Part model, mm, in its own coordinate system. A direction names the side the tool comes from. Coordinates: 2 decimals unless noted, no trailing zeros. Loops run counter-clockwise (first coordinate to the right, second up) from the corner with the lowest first, then second, coordinate; pieces in that order, holes last. Notation, with made-up numbers: M -15,36.5 L 28,36.5 A15 ccw 28,48.5 Z; hole C 33,24 d9. An arc over 180 degrees is marked long. Use a Markdown table: item, result. Add a question column.
1) Band-saw the part on C-C (x = -18.5). List the corners of the cut face in (y, z), plus the area to 3 significant figures.
2) Pull direction Z, two halves, no side cores. Call faces 5 (the flat face through (0, 1.2, 0)), 6 (the flat face through (22.5, 10, 0)), 7 (the flat face through (-11.5, 12, -23)): released by +Z, released by -Z, zero draft, split by the parting line, or undercut.
3) Band-saw the part on D-D (z = -0.5). List the corners of the cut face in (x, y), plus the area to 3 significant figures.
4) Band-saw the part on A-A (y = 13). List the corners of the cut face in (x, z).
5) Pin check, flat tips, straight feed: pin 1 Ø0.7 at (x, z) = (18.5, -18.5) entering from +Y; pin 2 Ø3 at (x, z) = (-18, -17.5) entering from +Y; pin 3 Ø1.3 at (x, z) = (-0.5, -23) entering from +Y. Stop position of each tip, or through.
6) Tool access for faces 1 (the cylindrical face through (-17.806, 3.721, 18.409)), 2 (the flat face through (-23, 12, 2)), 3 (the flat face through (11.5, 12, -23)), 4 (the flat face through (-9, 6.2, 23)): list every direction of +Z, -Z, +X, -X, +Y, -Y with a clear straight run to the whole face (end or side of a thin tool).
7) Band-saw the part on B-B (z = 10.5). List the corners of the cut face in (x, y).
8) Wall check: probe 1 along X at (y, z) = (3.6, -18.5); probe 2 along X at (y, z) = (4.75, -19); probe 3 along Z at (x, y) = (15, 15.25). Give the ranges that are in metal, low to high. Write a range as from..to.
from build123d import *

# Parameters (mm, degrees)
SKETCH1_W           = 47.4
SKETCH1_H           = 47.4
BOSS_EXTRUDE1_DEPTH = 18
SKETCH2_W           = 45
SKETCH2_H           = 45
CUT_EXTRUDE1_DEPTH  = 16.8
SKETCH3_R           = 1.75
BOSS_EXTRUDE2_DEPTH = 4
SKETCH4_R           = 0.7
CUT_EXTRUDE2_DEPTH  = 3
SKETCH5_W           = 16
SKETCH5_H           = 1.2
SKETCH5_W_2         = 1.2
SKETCH5_H_2         = 10.5
SKETCH5_W_3         = 23
CUT_EXTRUDE3_DEPTH  = 11.8


with BuildPart() as part:
    # Sketch1 → Boss-Extrude1 (new body)
    with BuildSketch(Plane(origin=(0, 0, 0), x_dir=(1, 0, 0), z_dir=(0, 1, 0))):
        Rectangle(SKETCH1_W, SKETCH1_H)
    extrude(amount=BOSS_EXTRUDE1_DEPTH)

    # Sketch2 → Cut-Extrude1 (cut)
    with BuildSketch(Plane(origin=(0, 18, 0), x_dir=(1, 0, 0), z_dir=(0, 1, 0))):
        Rectangle(SKETCH2_W, SKETCH2_H)
    extrude(amount=-CUT_EXTRUDE1_DEPTH, mode=Mode.SUBTRACT)

    # Sketch3 → Boss-Extrude2 (add)
    with BuildSketch(Plane(origin=(0, 1.2, 0), x_dir=(1, 0, 0), z_dir=(0, 1, 0))):
        with Locations(Location((-18.5, 18.5, 0), (0, 0, 270))):
            Circle(SKETCH3_R)
        with Locations(Location((18.5, 18.5, 0), (0, 0, 270))):
            Circle(SKETCH3_R)
        with Locations(Location((18.5, -18.5, 0), (0, 0, 270))):
            Circle(SKETCH3_R)
        with Locations(Location((-18.5, -18.5, 0), (0, 0, 270))):
            Circle(SKETCH3_R)
    extrude(amount=BOSS_EXTRUDE2_DEPTH)

    # Sketch4 → Cut-Extrude2 (cut)
    with BuildSketch(Plane(origin=(0, 5.2, 0), x_dir=(1, 0, 0), z_dir=(0, 1, 0))):
        with Locations(Location((-18.5, -18.5, 0), (0, 0, 270))):
            Circle(SKETCH4_R)
        with Locations(Location((-18.5, 18.5, 0), (0, 0, 270))):
            Circle(SKETCH4_R)
        with Locations(Location((18.5, 18.5, 0), (0, 0, 270))):
            Circle(SKETCH4_R)
        with Locations(Location((18.5, -18.5, 0), (0, 0, 270))):
            Circle(SKETCH4_R)
    extrude(amount=-CUT_EXTRUDE2_DEPTH, mode=Mode.SUBTRACT)

    # Sketch5 → Cut-Extrude3 (cut)
    with BuildSketch(Plane(origin=(0, 18, 0), x_dir=(1, 0, 0), z_dir=(0, 1, 0))):
        with Locations((-8.5, -23.1)):
            Rectangle(SKETCH5_W, SKETCH5_H)
        with Locations((23.1, -7.25)):
            Rectangle(SKETCH5_W_2, SKETCH5_H_2)
        with Locations((-23.1, -7.25)):
            Rectangle(SKETCH5_W_2, SKETCH5_H_2)
        with Locations((0, 23.1)):
            Rectangle(SKETCH5_W_3, SKETCH5_H)
    extrude(amount=-CUT_EXTRUDE3_DEPTH, mode=Mode.SUBTRACT)


solid = part.part
Entries:
| question | item | result |
|---|---|---|
| 1 | outline | M 0,-23.7 L 18,-23.7 L 18,-22.5 L 1.2,-22.5 L 1.2,-20.25 L 5.2,-20.25 L 5.2,-19.2 L 2.2,-19.2 L 2.2,-17.8 L 5.2,-17.8 L 5.2,-16.75 L 1.2,-16.75 L 1.2,16.75 L 5.2,16.75 L 5.2,17.8 L 2.2,17.8 L 2.2,19.2 L 5.2,19.2 L 5.2,20.25 L 1.2,20.25 L 1.2,22.5 L 18,22.5 L 18,23.7 L 0,23.7 Z |
| 1 | area | 117 mm2 |
| 2 | face 5 | undercut |
| 2 | face 6 | undercut |
| 2 | face 7 | zero draft |
| 3 | outline | M -23.7,0 L 23.7,0 L 23.7,18 L 22.5,18 L 22.5,1.2 L -22.5,1.2 L -22.5,18 L -23.7,18 Z |
| 3 | area | 97.2 mm2 |
| 4 | outline | M -23.7,-23.7 L -11.5,-23.7 L -11.5,-22.5 L -22.5,-22.5 L -22.5,2 L -23.7,2 Z; M -23.7,12.5 L -22.5,12.5 L -22.5,22.5 L -16.5,22.5 L -16.5,23.7 L -23.7,23.7 Z; M -0.5,22.5 L 22.5,22.5 L 22.5,12.5 L 23.7,12.5 L 23.7,23.7 L -0.5,23.7 Z; M 11.5,-23.7 L 23.7,-23.7 L 23.7,2 L 22.5,2 L 22.5,-22.5 L 11.5,-22.5 Z |
| 5 | pin 1 | y = 2.2 |
| 5 | pin 2 | y = 5.2 |
| 5 | pin 3 | y = 6.2 |
| 6 | face 1 | +Y |
| 6 | face 2 | +X, -X, +Y |
| 6 | face 3 | -Z, +Y |
| 6 | face 4 | +Z, +Y |
| 7 | outline | M -23.7,0 L 23.7,0 L 23.7,6.2 L 22.5,6.2 L 22.5,1.2 L -22.5,1.2 L -22.5,6.2 L -23.7,6.2 Z |
| 8 | probe 1 | -23.7..-22.5, -20.25..-19.2, -17.8..-16.75, 16.75..17.8, 19.2..20.25, 22.5..23.7 |
| 8 | probe 2 | -23.7..-22.5, -20.18..-18.99, -18.01..-16.82, 16.82..18.01, 18.99..20.18, 22.5..23.7 |
| 8 | probe 3 | -23.7..-22.5, 22.5..23.7 |
